from build123d import *

# Parameters (mm, degrees)
F0_W     = 63.5
F0_H     = 86.9489126992
F1_DEPTH = 63.5
F2_R     = 15.8444471424
F3_DEPTH = 49.1919759661
F4_W     = 21.8449309468
F4_H     = 30.9254080057
F5_DEPTH = 51.2255001813
F6_R     = 21.7743168909
F7_DEPTH = 135.4503948241


with BuildPart() as f1:
    # F0 (on Front) → F1 (new body)
    with BuildSketch(Plane.XZ):
        with Locations((31.75, 43.4744563496)):
            Rectangle(F0_W, F0_H)
    extrude(amount=F1_DEPTH)

    # F2 (on face) → F3 (join)
    with BuildSketch(Plane.XY.offset(86.9489126992)):
        with Locations((21.6802954674, -28.7499539554)):
            Circle(F2_R)
    extrude(amount=F3_DEPTH)

    # F4 (on face) → F5 (cut)
    with BuildSketch(Plane.YZ.offset(63.5)):
        with Locations((-23.2634544373, 44.0129265189)):
            Rectangle(F4_W, F4_H)
    extrude(amount=-F5_DEPTH, mode=Mode.SUBTRACT)

    # F6 (on face) → F7 (join)
    with BuildSketch(Plane.XZ.offset(63.5)):
        with Locations((33.4522090852, 42.7022464573)):
            Circle(F6_R)
    extrude(amount=F7_DEPTH)


solid = f1.part
Input: part model. Units: mm. Frame: model coordinates. A direction names the side the tool comes from. Coordinates: 2 decimals unless noted, no trailing zeros. Loops run counter-clockwise (first coordinate to the right, second up) from the corner with the lowest first, then second, coordinate; pieces in that order, holes last. Notation, with made-up numbers: (-26.75, 30.25) -> (-1.75, 30.25) arc R15 ccw to (-1.75, 49.25) -> close; hole circle Ø11 at (-23, 82.5). An arc over 180 degrees is marked (long way). One line per item, written item: value.
(1) Cut plane C-C (x = 53). Output: boundary loops of the cut face in (y, z), then the cut area to 3 significant figures.
Answer below:
outline: (-198.95, 33.11) -> (-63.5, 33.11) -> (-63.5, 0) -> (0, 0) -> (0, 86.95) -> (-63.5, 86.95) -> (-63.5, 52.29) -> (-198.95, 52.29) -> close; hole (-34.19, 28.55) -> (-12.34, 28.55) -> (-12.34, 59.48) -> (-34.19, 59.48) -> close
area: 7,440 mm2
(2) Draft query along Y for faces 1 (the face through (31, 0, 44)), 2 (the face through (38, -34.186, 44)), 3 (the face through (38, -23, 59.476)), 4 (the face through (33, -198.95, 43)). Return one class per face: pulls with the +Y half, pulls with the -Y half, needs draft (parallel to the pull), parting line crosses it, or undercut.
Answer below:
face 1: pulls with the +Y half
face 2: undercut
face 3: undercut
face 4: pulls with the -Y half
(3) Ray query, line 1 along Z through (x, y) = (36.5, -14); line 2 along Y through (x, z) = (40, 82.5); line 3 along Y through (x, z) = (50.5, 50). Return the intervals inside material, ascending.
Answer below:
line 1: z = 0 to 28.55, 59.48 to 86.95
line 2: y = -63.5 to 0
line 3: y = -198.95 to -34.19, -12.34 to 0
(4) Cut plane B-B (z = 36.5). Output: boundary loops of the cut face in (x, y).
Answer below:
outline: (0, -63.5) -> (12.58, -63.5) -> (12.58, -198.95) -> (54.32, -198.95) -> (54.32, -63.5) -> (63.5, -63.5) -> (63.5, -34.19) -> (12.27, -34.19) -> (12.27, -12.34) -> (63.5, -12.34) -> (63.5, 0) -> (0, 0) -> close
(5) Cut plane A-A (x = 22). Output: boundary loops of the cut face in (y, z).
Answer below:
outline: (-198.95, 24.18) -> (-63.5, 24.18) -> (-63.5, 0) -> (0, 0) -> (0, 86.95) -> (-12.91, 86.95) -> (-12.91, 136.14) -> (-44.59, 136.14) -> (-44.59, 86.95) -> (-63.5, 86.95) -> (-63.5, 61.22) -> (-198.95, 61.22) -> close; hole (-34.19, 28.55) -> (-12.34, 28.55) -> (-12.34, 59.48) -> (-34.19, 59.48) -> close
(6) Set-up query: faces 5 (the face through (12.274, -23, 44)), 6 (the face through (24, -63.5, 63)), 7 (the face through (36.793, -23.991, 111.201)). Return all of +Z, -Z, +X, -X, +Y, -Y with unobstructed straight access to the full face (end or side cutting, diameter ignored); none if empty.
Answer below:
face 5: +X
face 6: -Y
face 7: +Z
(7) Cut plane D-D (z = 12). Output: boundary loops of the cut face in (x, y), then the cut area to 3 significant figures.
Answer below:
outline: (0, -63.5) -> (63.5, -63.5) -> (63.5, 0) -> (0, 0) -> close
area: 4,030 mm2
(8) Pin query (flat end, axial travel): pin 1 Ø12 at (x, y) = (25.5, -143.5) entering from +Z; pin 2 Ø5 at (x, z) = (36, 112.5) entering from -Y; pin 3 Ø2 at (x, y) = (47, -149) entering from -Z. Return the tip coordinate at first contact, or that it passes through.
Answer below:
pin 1: stops at z = 64.39
pin 2: stops at y = -39.3
pin 3: stops at z = 24.91
